Input: part model. Units: mm. Frame: model coordinates. Face numbers are marked on the shaded views. A direction names the side the tool comes from. Coordinates: 2 decimals unless noted, no trailing zeros. Order: outer loops, then holes, each group sorted by start corner. A loop starts at its lowest first (then second) coordinate and runs counter-clockwise, first axis right, second up. Notation, with made-up numbers: (20.25, -25) -> (73.25, -25) arc R19 ccw to (73.25, -13) -> close; hole circle Ø3 at (81.5, 66.25). An arc over 180 degrees is marked (long way). Answer as CSV lines item,"result".
from build123d import *

# Parameters (mm, degrees)
SKETCH1_W           = 30
SKETCH1_H           = 8
SKETCH1_R           = 1.55
BOSS_EXTRUDE1_DEPTH = 6
SKETCH6_W           = 50
SKETCH6_H           = 24
BOSS_EXTRUDE4_DEPTH = 12
SKETCH8_W           = 11
SKETCH8_H           = 8
CUT_EXTRUDE2_DEPTH  = 8
FILLET1_R           = 1
FILLET2_R           = 1
CHAMFER2_SIZE       = 0.6
CHAMFER3_SIZE       = 0.5


with BuildPart() as part:
    # Sketch1 → Boss-Extrude1 (new, symmetric)
    with BuildSketch(Plane.XY):
        Rectangle(SKETCH1_W, SKETCH1_H)
        with Locations((10, 0)):
            Circle(SKETCH1_R, mode=Mode.SUBTRACT)
        with Locations(Location((-10, 0, 0), (0, 0, 180))):
            Circle(SKETCH1_R, mode=Mode.SUBTRACT)
    extrude(amount=BOSS_EXTRUDE1_DEPTH, both=True)

    # Sketch6 → Boss-Extrude4 (add)
    with BuildSketch(Plane(origin=(0, 0, -6), x_dir=(-1, 0, 0), z_dir=(0, 0, -1))):
        with Locations((0, 16)):
            Rectangle(SKETCH6_W, SKETCH6_H)
    extrude(amount=-BOSS_EXTRUDE4_DEPTH)

    # Sketch8 → Cut-Extrude2 (cut)
    with BuildSketch(Plane(origin=(0, 0, -6), x_dir=(-1, 0, 0), z_dir=(0, 0, -1))):
        Rectangle(SKETCH8_W, SKETCH8_H)
        Polygon((-23, 25), (-23, 4), (-15, 4), (-5.5, 4), (5.5, 4), (15, 4), (23, 4), (23, 25), align=None)
    extrude(amount=-CUT_EXTRUDE2_DEPTH, mode=Mode.SUBTRACT)

    # Fillet1
    fillet1_edges = [part.edges().sort_by_distance(p)[0] for p in [
        (25, 16, 6),
        (0, 28, 6),
        (-25, 16, 6),
    ]]
    fillet(fillet1_edges, radius=FILLET1_R)

    # Fillet2
    # the kernel refuses this fillet: 1 mm, written as the material it takes off along each edge
    with BuildSketch(Plane(origin=(24, 27, 5), x_dir=(0, 1, 0), z_dir=(1, 0, 0))) as fillet2_piece_1_section:
        Polygon((0, 0), (FILLET2_R, 0), (FILLET2_R, FILLET2_R), (0, FILLET2_R), align=None)
    fillet2_piece_1 = extrude(amount=FILLET2_R, mode=Mode.PRIVATE)
    fillet2_piece_1 = fillet2_piece_1 - Plane(origin=(24, 27, 5), x_dir=(0, -0.7071067811865475, -0.7071067811865475), z_dir=(1, 0, 0)) * Sphere(FILLET2_R, mode=Mode.PRIVATE)
    add(fillet2_piece_1, mode=Mode.SUBTRACT)
    with BuildSketch(Plane(origin=(-24, 27, 5), x_dir=(-1, 0, 0), z_dir=(0, 1, 0))) as fillet2_piece_2_section:
        Polygon((0, 0), (FILLET2_R, 0), (FILLET2_R, FILLET2_R), (0, FILLET2_R), align=None)
    fillet2_piece_2 = extrude(amount=FILLET2_R, mode=Mode.PRIVATE)
    fillet2_piece_2 = fillet2_piece_2 - Plane(origin=(-24, 27, 5), x_dir=(0.7071067811865475, 0, -0.7071067811865475), z_dir=(0, 1, 0)) * Sphere(FILLET2_R, mode=Mode.PRIVATE)
    add(fillet2_piece_2, mode=Mode.SUBTRACT)
    with BuildSketch(Plane(origin=(-15, 4, 6), x_dir=(1, 0, 0), z_dir=(0, -1, 0)), Plane(origin=(15, -6.5, 6), x_dir=(-1, 0, 0), z_dir=(0, 1, 0))) as fillet2_piece_3:
        with BuildLine():
            CenterArc((FILLET2_R, -FILLET2_R), FILLET2_R, 90, 90)
            Line((0, -FILLET2_R), (0, 0))
            Line((0, 0), (FILLET2_R, 0))
        make_face()
    extrude(amount=10.5, mode=Mode.SUBTRACT)
    with BuildSketch(Plane(origin=(-17.5, -4, 6), x_dir=(0, 1, 0), z_dir=(1, 0, 0))) as fillet2_piece_4:
        with BuildLine():
            CenterArc((FILLET2_R, -FILLET2_R), FILLET2_R, 90, 90)
            Line((0, -FILLET2_R), (0, 0))
            Line((0, 0), (FILLET2_R, 0))
        make_face()
    extrude(amount=35, mode=Mode.SUBTRACT)
    with BuildSketch(Plane(origin=(24, 4, 6), x_dir=(0, 0, -1), z_dir=(-1, 0, 0))) as fillet2_piece_5:
        with BuildLine():
            CenterArc((FILLET2_R, -FILLET2_R), FILLET2_R, 90, 90)
            Line((0, -FILLET2_R), (0, 0))
            Line((0, 0), (FILLET2_R, 0))
        make_face()
    extrude(amount=9, mode=Mode.SUBTRACT)
    with BuildSketch(Plane(origin=(-15, 4, 6), x_dir=(0, 1, 0), z_dir=(-1, 0, 0))) as fillet2_piece_6:
        with BuildLine():
            CenterArc((FILLET2_R, FILLET2_R), FILLET2_R, 180, 90)
            Line((0, FILLET2_R), (0, 0))
            Line((0, 0), (FILLET2_R, 0))
        make_face()
    extrude(amount=9, mode=Mode.SUBTRACT)
    with BuildSketch(Plane(origin=(-25, 4, -8.5), x_dir=(1, 0, 0), z_dir=(0, 0, 1))) as fillet2_piece_7:
        with BuildLine():
            CenterArc((FILLET2_R, FILLET2_R), FILLET2_R, 180, 90)
            Line((0, FILLET2_R), (0, 0))
            Line((0, 0), (FILLET2_R, 0))
        make_face()
    extrude(amount=13.5, mode=Mode.SUBTRACT)
    with BuildSketch(Plane(origin=(-24, 4, 5), x_dir=(0, 0, 1), z_dir=(1, 0, 0))) as fillet2_piece_8:
        with BuildLine():
            CenterArc((1 - FILLET2_R, -FILLET2_R), FILLET2_R, 0, 90)
            Line((1 - FILLET2_R, 0), (1, 0))
            Line((1, 0), (1, -FILLET2_R))
        make_face()
    revolve(axis=Axis((-24, 4, 5), (0, -1, 0)), revolution_arc=90, mode=Mode.SUBTRACT)
    with BuildSketch(Plane(origin=(-25, 28, -8.5), x_dir=(1, 0, 0), z_dir=(0, 0, 1)), Plane(origin=(25, 4, -8.5), x_dir=(-1, 0, 0), z_dir=(0, 0, 1)), Plane(origin=(25, 28, -8.5), x_dir=(0, -1, 0), z_dir=(0, 0, 1))) as fillet2_piece_9:
        with BuildLine():
            CenterArc((FILLET2_R, -FILLET2_R), FILLET2_R, 90, 90)
            Line((0, -FILLET2_R), (0, 0))
            Line((0, 0), (FILLET2_R, 0))
        make_face()
    extrude(amount=13.5, mode=Mode.SUBTRACT)
    with BuildSketch(Plane(origin=(24, 4, 5), x_dir=(0, 0, 1), z_dir=(-1, 0, 0))) as fillet2_piece_10:
        with BuildLine():
            CenterArc((1 - FILLET2_R, FILLET2_R), FILLET2_R, 270, 90)
            Line((1, FILLET2_R), (1, 0))
            Line((1, 0), (1 - FILLET2_R, 0))
        make_face()
    revolve(axis=Axis((24, 4, 5), (0, 1, 0)), revolution_arc=90, mode=Mode.SUBTRACT)
    with BuildSketch(Plane(origin=(-15, 6.5, 6), x_dir=(1, 0, 0), z_dir=(0, -1, 0))) as fillet2_piece_11a_section:
        with BuildLine():
            CenterArc((FILLET2_R, -FILLET2_R), FILLET2_R, 90, 90)
            Line((0, -FILLET2_R), (0, 0))
            Line((0, 0), (FILLET2_R, 0))
        make_face()
    fillet2_piece_11a = extrude(amount=13, mode=Mode.PRIVATE)
    fillet2_piece_11a = split(fillet2_piece_11a, bisect_by=Plane(origin=(-14.773604886, 4, 5.773604886), z_dir=(0, 1, 0)), keep=Keep.TOP, mode=Mode.PRIVATE)
    with BuildSketch(Plane(origin=(-12.5, 4, 6), x_dir=(0, 1, 0), z_dir=(-1, 0, 0))) as fillet2_piece_11b_section:
        with BuildLine():
            CenterArc((FILLET2_R, FILLET2_R), FILLET2_R, 180, 90)
            Line((0, FILLET2_R), (0, 0))
            Line((0, 0), (FILLET2_R, 0))
        make_face()
    fillet2_piece_11b = extrude(amount=11.5, mode=Mode.PRIVATE)
    fillet2_piece_11b = split(fillet2_piece_11b, bisect_by=Plane(origin=(-15, 4.226395114, 5.773604886), z_dir=(1, 0, 0)), keep=Keep.TOP, mode=Mode.PRIVATE)
    fillet2_piece_11 = fillet2_piece_11a & fillet2_piece_11b
    add(fillet2_piece_11, mode=Mode.SUBTRACT)
    with BuildSketch(Plane(origin=(24, 4, 6), x_dir=(0, 0, -1), z_dir=(-1, 0, 0))) as fillet2_piece_12a_section:
        with BuildLine():
            CenterArc((FILLET2_R, -FILLET2_R), FILLET2_R, 90, 90)
            Line((0, -FILLET2_R), (0, 0))
            Line((0, 0), (FILLET2_R, 0))
        make_face()
    fillet2_piece_12a = extrude(amount=11.5, mode=Mode.PRIVATE)
    fillet2_piece_12a = split(fillet2_piece_12a, bisect_by=Plane(origin=(15, 4.226395114, 5.773604886), z_dir=(-1, 0, 0)), keep=Keep.TOP, mode=Mode.PRIVATE)
    with BuildSketch(Plane(origin=(15, -6.5, 6), x_dir=(-1, 0, 0), z_dir=(0, 1, 0))) as fillet2_piece_12b_section:
        with BuildLine():
            CenterArc((FILLET2_R, -FILLET2_R), FILLET2_R, 90, 90)
            Line((0, -FILLET2_R), (0, 0))
            Line((0, 0), (FILLET2_R, 0))
        make_face()
    fillet2_piece_12b = extrude(amount=13, mode=Mode.PRIVATE)
    fillet2_piece_12b = split(fillet2_piece_12b, bisect_by=Plane(origin=(14.773604886, 4, 5.773604886), z_dir=(0, 1, 0)), keep=Keep.TOP, mode=Mode.PRIVATE)
    fillet2_piece_12 = fillet2_piece_12a & fillet2_piece_12b
    add(fillet2_piece_12, mode=Mode.SUBTRACT)

    # Chamfer2
    chamfer2_edges = [part.edges().sort_by_distance(p)[0] for p in [
        (-25, 16, -6),
        (0, 28, -6),
        (25, 16, -6),
        (24.707106781, 27.707106781, -6),
        (-24.707106781, 27.707106781, -6),
        (24.707106781, 4.292893219, -6),
        (-24.707106781, 4.292893219, -6),
        (-23.5, 4, -6),
        (23.5, 4, -6),
    ]]
    chamfer(chamfer2_edges, length=CHAMFER2_SIZE)

    # Chamfer3
    chamfer3_edges = [part.edges().sort_by_distance(p)[0] for p in [
        (8.45, 0, -6),
        (-8.45, 0, -6),
        (10.25, -4, -6),
        (-5.5, 0, -6),
        (-10.25, -4, -6),
        (-15, 0, -6),
        (-10.25, 4, -6),
        (10.25, 4, -6),
        (5.5, 0, -6),
        (15, 0, -6),
    ]]
    chamfer(chamfer3_edges, length=CHAMFER3_SIZE)


solid = part.part
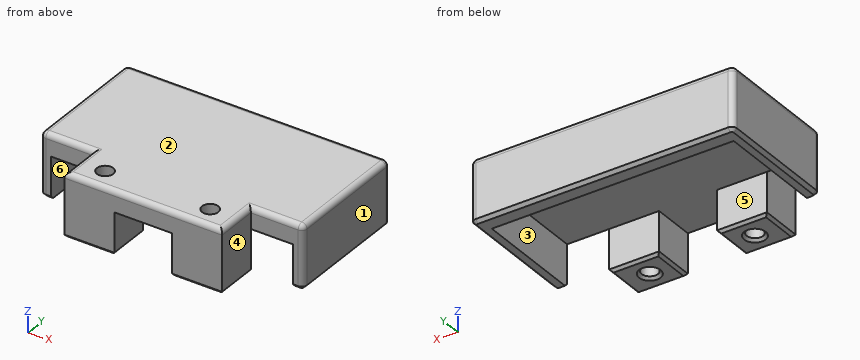
1. Contact query for flat-ended pins moving along their axis: pin 1 (4 mm diameter, centred on y = 0, z = -2, fed in from -X); pin 2 (2.5 mm diameter, centred on x = 10, y = 0, fed in from -Z); pin 3 (8.5 mm diameter, centred on x = -1.5, y = 17.5, fed in from -Z); pin 4 (4 mm diameter, centred on y = 0, z = -1.5, fed in from +X). Output: stop coordinate, or through.
Findings:
pin 1,"stops at x = -15"
pin 2,"passes through"
pin 3,"stops at z = 2"
pin 4,"stops at x = 15"
2. Ray query, line 1 along Y through (x, z) = (-10, 0.5); line 2 along X through (y, z) = (19, -2); line 3 along Y through (x, z) = (10, 3.75). Return the intervals inside material, ascending.
Findings:
line 1,"y = -4 to -1.55, 1.55 to 4, 25 to 28"
line 2,"x = -25 to -23, 23 to 25"
line 3,"y = -4 to -1.55, 1.55 to 28"
3. Cut plane C-C (x = -10). Return the cut outline in (y, z).
Findings:
outline,"(-4, -5.5) -> (-3.5, -6) -> (-2.05, -6) -> (-1.55, -5.5) -> (-1.55, 6) -> (-3, 6) arc R1 ccw to (-4, 5) -> close; (1.55, -5.5) -> (2.05, -6) -> (3.5, -6) -> (4, -5.5) -> (4, 2) -> (25, 2) -> (25, -6) -> (27.4, -6) -> (28, -5.4) -> (28, 5) arc R1 ccw to (27, 6) -> (1.55, 6) -> close"
4. Cut plane B-B (y = 0). Return the cut outline in (x, z).
Findings:
outline,"(-15, -5.5) -> (-14.5, -6) -> (-12.05, -6) -> (-11.55, -5.5) -> (-11.55, 6) -> (-14, 6) arc R1 ccw to (-15, 5) -> close; (-8.45, -5.5) -> (-7.95, -6) -> (-6, -6) -> (-5.5, -5.5) -> (-5.5, 2) -> (5.5, 2) -> (5.5, -5.5) -> (6, -6) -> (7.95, -6) -> (8.45, -5.5) -> (8.45, 6) -> (-8.45, 6) -> close; (11.55, -5.5) -> (12.05, -6) -> (14.5, -6) -> (15, -5.5) -> (15, 5) arc R1 ccw to (14, 6) -> (11.55, 6) -> close"
5. Cut plane A-A (z = -4.25). Return the cut outline in (x, y).
Findings:
outline,"(-25, 5) arc R1 ccw to (-24, 4) -> (-23, 4) -> (-23, 25) -> (23, 25) -> (23, 4) -> (24, 4) arc R1 ccw to (25, 5) -> (25, 27) arc R1 ccw to (24, 28) -> (-24, 28) arc R1 ccw to (-25, 27) -> close; (-15, -4) -> (-5.5, -4) -> (-5.5, 4) -> (-15, 4) -> close; (5.5, -4) -> (15, -4) -> (15, 4) -> (5.5, 4) -> close; hole circle Ø3.1 at (-10, 0); hole circle Ø3.1 at (10, 0)"
6. Cut plane D-D (x = -21). Return the cut outline in (y, z).
Findings:
outline,"(4, 2) -> (25, 2) -> (25, -6) -> (27.4, -6) -> (28, -5.4) -> (28, 5) arc R1 ccw to (27, 6) -> (5, 6) arc R1 ccw to (4, 5) -> close"
7. Reachability of the marked faces 4, 5 and 6 from +Z, -Z, +X, -X, +Y, -Y: full face, straight path, thin tool, end or side. Return the list, or none.
Findings:
face 4,"+Z, -Z, +X, -Y"
face 5,"-Z"
face 6,"-Z, -Y"
8. Mould query, pull axis X, two halves, no side actions, for the marked faces 1, 2 and 3. Classes: released by +X, released by -X, zero draft, split by the parting line, or undercut.
Findings:
face 1,"released by +X"
face 2,"zero draft"
face 3,"undercut"
